Job drawing, mm, ordinate dimensions from the low corner. One solid piece. A direction names the side the tool comes from. Coordinates: 2 decimals unless noted, no trailing zeros. Order: outer loops, then holes, each group sorted by start corner. A loop starts at its lowest first (then second) coordinate and runs counter-clockwise, first axis right, second up. Notation, with made-up numbers: (16.5, 21) - (27.5, 21) arc R5 ccw to (27.5, 25) - close; hole circle Ø5 at (55.25, 87.5). An arc over 180 degrees is marked (long way). Use a Markdown table: item, result. Add a question column.
1) Saw through at D-D on x = 9.5. List the corners of the cut face in (y, z) (3 decimals).
2) Wall check: L1, parallel to Z at x = 4.5, y = 5.75; L2, parallel to Z at x = 5.5, y = 7.5; L3, parallel to X at y = 2.75, z = 5.25 (1 decimal). Give the ranges that are in metal, low to high. Write a range as [from, to].
3) Drop flat-ended pins along their axis: P1, Ø0.5, axis at y = 4.5, z = 7.5, coming from the +X side; P2, Ø3.5, axis at x = 2.5, y = 5.5, coming from the -Z side; P3, Ø2.5, axis at x = 4.64, y = 4, coming from the -Z side. Give the stop position or say it passes through.
4) Saw through at C-C on x = 4. List the corners of the cut face in (y, z).
5) Tool access for the marked faces 4, 5 and 6: list every direction of +Z, -Z, +X, -X, +Y, -Y with a clear straight run to the whole face (end or side of a thin tool).
6) Saw through at A-A on z = 6. List the corners of the cut face in (x, y) (1 decimal), then the cut area to 3 significant figures.
7) Two-plate mould, pull along Y, no slides. Class the marked faces 1, 2 and 3: +Y half, -Y half, draft (parallel to the pull), parting line (faces both ways), or undercut.
8) Saw through at B-B on y = 4. List the corners of the cut face in (x, z) (3 decimals), then the cut area to 3 significant figures.
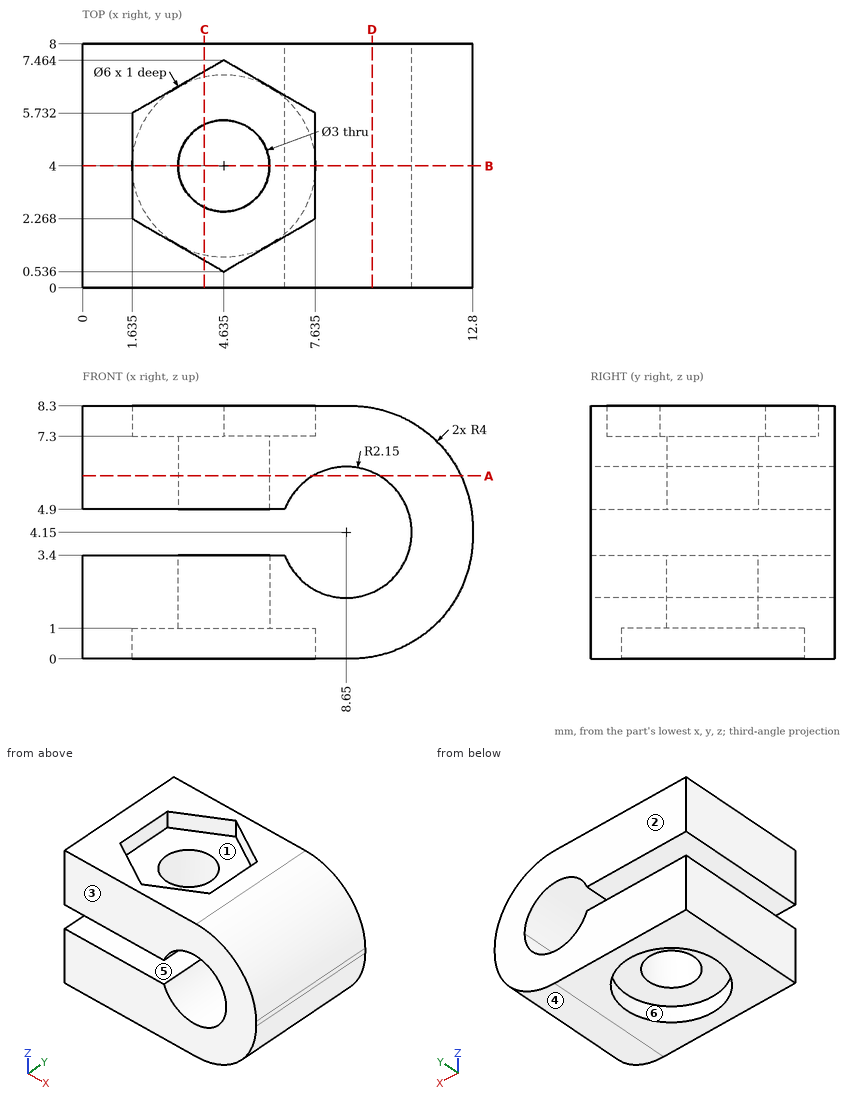
Results are:
| question | item | result |
|---|---|---|
| 1 | outline | (0, 0.062) - (8, 0.062) - (8, 2.175) - (0, 2.175) - close; (0, 6.125) - (8, 6.125) - (8, 8.238) - (0, 8.238) - close |
| 2 | L1 | [1, 3.4], [4.9, 7.3] |
| 2 | L2 | [0, 3.4], [4.9, 8.3] |
| 2 | L3 | [0, 3.8], [5.5, 6.8], [10.5, 12.7] |
| 3 | P1 | x = 11.5 |
| 3 | P2 | z = 0 |
| 3 | P3 | through |
| 4 | outline | (0, 0) - (1.07, 0) - (1.07, 1) - (2.64, 1) - (2.64, 3.4) - (0, 3.4) - close; (0, 4.9) - (2.64, 4.9) - (2.64, 7.3) - (0.9, 7.3) - (0.9, 8.3) - (0, 8.3) - close; (5.36, 1) - (6.93, 1) - (6.93, 0) - (8, 0) - (8, 3.4) - (5.36, 3.4) - close; (5.36, 4.9) - (8, 4.9) - (8, 8.3) - (7.1, 8.3) - (7.1, 7.3) - (5.36, 7.3) - close |
| 5 | face 4 | -Z, +X, +Y, -Y |
| 5 | face 5 | -X, +Y, -Y |
| 5 | face 6 | -Z |
| 6 | outline | (0, 0) - (7.6, 0) - (7.6, 8) - (0, 8) - close; (9.7, 0) - (12.4, 0) - (12.4, 8) - (9.7, 8) - close; hole circle Ø3 at (4.6, 4) |
| 6 | area | 74.8 mm2 |
| 7 | face 1 | undercut |
| 7 | face 2 | +Y half |
| 7 | face 3 | -Y half |
| 8 | outline | (0, 0) - (1.635, 0) - (1.635, 1) - (3.135, 1) - (3.135, 3.4) - (0, 3.4) - close; (0, 4.9) - (3.135, 4.9) - (3.135, 7.3) - (1.635, 7.3) - (1.635, 8.3) - (0, 8.3) - close; (6.135, 1) - (7.635, 1) - (7.635, 0) - (8.8, 0) arc R4 ccw to (12.8, 4) - (12.8, 4.3) arc R4 ccw to (8.8, 8.3) - (7.635, 8.3) - (7.635, 7.3) - (6.135, 7.3) - (6.135, 4.9) - (6.635, 4.9) arc R2.15 cw (long way) to (6.635, 3.4) - (6.135, 3.4) - close |
| 8 | area | 48.6 mm2 |
